Autodesk Inventor part; units mm, degrees
ref_plane "YZ Plane" through (0, 0, 0) normal (1, 0, 0) x (0, 1, 0)
ref_plane "XZ Plane" through (0, 0, 0) normal (0, 1, 0) x (-1, 0, 0)
ref_plane "XY Plane" through (0, 0, 0) normal (0, 0, 1) x (1, 0, 0)
sketch "스케치1" plane through (0, 0, 0) normal (0, 1, 0) x (-1, 0, 0)
  line L0 (0, 0) -> (11, 0)
  line L1 (11, 0) -> (11, -4)
  line L2 (11, -4) -> (0, -4)
  line L3 (0, -4) -> (0, 0)
  dimension "d0" = 11
  dimension "d1" = 4
extrude "돌출1" add sketch "스케치1" along normal blind 7
sketch "스케치2" plane through (0, 7, 0) normal (0, 1, 0) x (1, 0, 0)
  line L0 (0, 0) -> (0, 4) construction
  line L1 (0, 2) -> (-11, 2) construction
  line L2 (-11, 4) -> (-11, 0) construction
  point P0 (-1.3, 2)
  point P1 (-4.3, 2)
  point P2 (-7.5, 2)
  point P3 (-9.7, 2)
  point P4 (-4.3, 2)
  dimension "d59" = 1.3
  dimension "d60" = 2.2
  dimension "d61" = 3.2
  dimension "d62" = 1.3
  dimension "d69" = 0
hole "구멍1" at (-9.7, 7, -2) at (-1.3, 7, -2) direction (0, -1, 0) diameter 0.65 end through all
hole "구멍2" at (-7.5, 7, -2) direction (0, -1, 0) diameter 1.3 end through all
hole "구멍3" at (-4.3, 7, -2) direction (0, -1, 0) diameter 0.67 end through all
sketch "스케치3" plane through (0, 7, 0) normal (0, 1, 0) x (1, 0, 0)
  circle A0 centre (-4.3, 2) radius 1
  circle A1 centre (-4.3, 2) radius 0.335
  point P0 (0, 0)
  point P1 (-4.3, 2)
  dimension "d50" = 2
extrude "돌출2" add sketch "스케치3" along normal blind 1.5
sketch "스케치4" plane through (0, 0, 0) normal (0, -1, 0) x (1, 0, 0)
  circle A0 centre (-4.3, -2) radius 1
  circle A1 centre (-4.3, -2) radius 0.335
  point P0 (0, 0)
  point P1 (-4.3, -2)
  dimension "d53" = 2
extrude "돌출3" add sketch "스케치4" along normal blind 1.5
equation "\"d8\" = G23_F"
equation "\"d15\" = Screw_F"
equation "\"d22\" = G23_M"
equation "\"G23_F\" = 0.65"
equation "\"G23_M\" = 0.67"
equation "\"Screw_F\" = 1.3"
equation "\"Screw_M\" = 1.6"
properties part number "_3D 인쇄"
Read the model definition and answer for the solid it produces. Units are mm, in the model's axes. A direction names the side the tool comes from. Round coordinates to 2 decimals unless told otherwise and drop trailing zeros. Order: outer loops, then holes, each group sorted by start corner. A loop starts at its lowest first (then second) coordinate and runs counter-clockwise, first axis right, second up.
1) The part is cut by section B-B on z = -2. Write down the section's boundary in (x, y) (3 decimals), plus the area to 3 significant figures.
2) For faces 1 (the face through (-11, 3, -2)), 2 (the face through (-5.1, 7.7, -2.6)), 3 (the face through (-4.517, -0.74, -1.024)), determine the directions among +Z, -Z, +X, -X, +Y, -Y from which every point of the face is accessible in a straight line to the end or side of a thin tool.
3) The part is cut by section D-D on x = -7.5. Write down the section's boundary in (y, z).
4) The part is cut by section C-C on y = 0.5. Write down the section's boundary in (x, z) (3 decimals), plus the area to 3 significant figures.
5) Flat-ended cylindrical pins translate along their axes: pin 1 (1 mm diameter, centred on x = -1.5, z = -1.5, fed in from -Y); pin 2 (2 mm diameter, centred on x = -9.5, z = -2, fed in from +Y). Find the tip coordinate at first contact, or state that the pin passes through.
6) Straight lines are drawn through the part: L1, parallel to X at y = 3, z = -2 (3 decimals); L2, parallel to Z at x = -1.3, y = 5 (3 decimals); L3, parallel to Z at x = -7.5, y = 5. For each, find the intervals that lie inside material, in ascending order.
7) The part is cut by section A-A on x = -4.3. Write down the section's boundary in (y, z) (3 decimals).
8) The mould has two halves that part along Z. Classify faces 4 (the face through (-6, 3, -4)), 5 (the face through (-8.05, 3.45, -1.65)), 6 (the face through (-4.3, -1.5, -1.5)): released by +Z, released by -Z, zero draft, split by the parting line, or undercut.
Resolved:
1. outline: (-11, 0) - (-10.025, 0) - (-10.025, 7) - (-11, 7) - close; (-9.375, 0) - (-8.15, 0) - (-8.15, 7) - (-9.375, 7) - close; (-6.85, 0) - (-5.3, 0) - (-5.3, -1.5) - (-4.635, -1.5) - (-4.635, 8.5) - (-5.3, 8.5) - (-5.3, 7) - (-6.85, 7) - close; (-3.965, -1.5) - (-3.3, -1.5) - (-3.3, 0) - (-1.625, 0) - (-1.625, 7) - (-3.3, 7) - (-3.3, 8.5) - (-3.965, 8.5) - close; (-0.975, 0) - (0, 0) - (0, 7) - (-0.975, 7) - close
1. area: 58.1 mm2
2. face 1: +Z, -Z, -X, +Y, -Y
2. face 2: +Y
2. face 3: -Y
3. outline: (0, -4) - (7, -4) - (7, -2.65) - (0, -2.65) - close; (0, -1.35) - (7, -1.35) - (7, 0) - (0, 0) - close
4. outline: (-11, -4) - (0, -4) - (0, 0) - (-11, 0) - close; hole circle Ø0.65 at (-9.7, -2); hole circle Ø1.3 at (-7.5, -2); hole circle Ø0.67 at (-4.3, -2); hole circle Ø0.65 at (-1.3, -2)
4. area: 41.7 mm2
5. pin 1: stops at y = 0
5. pin 2: stops at y = 7
6. L1: x = -11 to -10.025, -9.375 to -8.15, -6.85 to -4.635, -3.965 to -1.625, -0.975 to 0
6. L2: z = -4 to -2.325, -1.675 to 0
6. L3: z = -4 to -2.65, -1.35 to 0
7. outline: (-1.5, -3) - (0, -3) - (0, -4) - (7, -4) - (7, -3) - (8.5, -3) - (8.5, -2.335) - (-1.5, -2.335) - close; (-1.5, -1.665) - (8.5, -1.665) - (8.5, -1) - (7, -1) - (7, 0) - (0, 0) - (0, -1) - (-1.5, -1) - close
8. face 4: released by -Z
8. face 5: undercut
8. face 6: zero draft
